The listing builds one solid part. Answer for the finished solid, in the listing's coordinates (mm). A direction names the side the tool comes from. Coordinates: 2 decimals unless noted, no trailing zeros. Order: outer loops, then holes, each group sorted by start corner. A loop starts at its lowest first (then second) coordinate and runs counter-clockwise, first axis right, second up. Notation, with made-up numbers: (52.5, -22) -> (62.5, -22) arc R9 ccw to (62.5, -8) -> close; hole circle Ø5 at (51.5, 25). An arc over 180 degrees is marked (long way). Put each result on its own line as item: value. Start each with the question number.
```python
from build123d import *

# Parameters (mm, degrees)
SKETCH1_R           = 19
SKETCH1_R_2         = 10.2
BOSS_EXTRUDE1_DEPTH = 5
SKETCH2_R           = 1.5
CUT_EXTRUDE1_DEPTH  = 5
BOSS_EXTRUDE2_START = -5
BOSS_EXTRUDE2_DEPTH = 5
SKETCH7_W           = 25
SKETCH7_H           = 5
BOSS_EXTRUDE5_DEPTH = 20
SKETCH8_W           = 20
SKETCH8_H           = 50
BOSS_EXTRUDE6_DEPTH = 5
SKETCH9_W           = 20
SKETCH9_H           = 50
BOSS_EXTRUDE7_DEPTH = 5


with BuildPart() as part:
    # Sketch1 → Boss-Extrude1 (new body)
    with BuildSketch(Plane(origin=(0, 0, 0), x_dir=(1, 0, 0), z_dir=(0, 1, 0))):
        with Locations(Location((0, 0, 0), (0, 0, 270))):
            Circle(SKETCH1_R)
        with Locations(Location((0, 0, 0), (0, 0, 270))):
            Circle(SKETCH1_R_2, mode=Mode.SUBTRACT)
    extrude(amount=BOSS_EXTRUDE1_DEPTH)

    # Sketch2 → Cut-Extrude1 (cut)
    with BuildSketch(Plane(origin=(0, 5, 0), x_dir=(1, 0, 0), z_dir=(0, 1, 0))):
        with Locations(Location((0, 14, 0), (0, 0, 270))):
            Circle(SKETCH2_R)
        with Locations(Location((7.5, 12.990381057, 0), (0, 0, 270))):
            Circle(SKETCH2_R)
        with Locations(Location((12.124355653, -7, 0), (0, 0, 270))):
            Circle(SKETCH2_R)
        with Locations(Location((7.5, -12.990381057, 0), (0, 0, 270))):
            Circle(SKETCH2_R)
        with Locations(Location((-12.124355653, -7, 0), (0, 0, 270))):
            Circle(SKETCH2_R)
        with Locations(Location((-15, 0, 0), (0, 0, 270))):
            Circle(SKETCH2_R)
    extrude(amount=-CUT_EXTRUDE1_DEPTH, mode=Mode.SUBTRACT)

    # Sketch3 → Boss-Extrude2 (add)
    with BuildSketch(Plane(origin=(0, 5, 0), x_dir=(1, 0, 0), z_dir=(0, 1, 0)).offset(BOSS_EXTRUDE2_START)):
        with BuildLine():
            ThreePointArc((19, 0), (13.435028843, -13.435028843), (0, -19))
            Line((0, -19), (23, -19))
            Line((23, -19), (23, 19))
            Line((23, 19), (0, 19))
            ThreePointArc((0, 19), (13.435028843, 13.435028843), (19, 0))
        make_face()
    extrude(amount=BOSS_EXTRUDE2_DEPTH)

    # Sketch7 → Boss-Extrude5 (add)
    with BuildSketch(Plane(origin=(23, 0, 0), x_dir=(0, 0, -1), z_dir=(1, 0, 0))):
        with Locations((0, 2.5)):
            Rectangle(SKETCH7_W, SKETCH7_H)
    extrude(amount=BOSS_EXTRUDE5_DEPTH)

    # Sketch8 → Boss-Extrude6 (add)
    with BuildSketch(Plane.XY.offset(12.5)):
        with Locations((33, -20)):
            Rectangle(SKETCH8_W, SKETCH8_H)
    extrude(amount=-BOSS_EXTRUDE6_DEPTH)

    # Sketch9 → Boss-Extrude7 (add)
    with BuildSketch(Plane(origin=(0, 0, -12.5), x_dir=(-1, 0, 0), z_dir=(0, 0, -1))):
        with Locations((-33, -20)):
            Rectangle(SKETCH9_W, SKETCH9_H)
    extrude(amount=-BOSS_EXTRUDE7_DEPTH)


solid = part.part
```
(1) For a pull along Z with two mould halves and no side action, classify faces 6 (the flat face through (11, 2, 19)), 7 (the cylindrical face through (6.587, 2.535, -14.181)), 8 (the flat face through (12, 2, -19)) as released by +Z, released by -Z, zero draft, split by the parting line, or undercut.
(2) Find the intervals of material crossed by L1, parallel to X at y = 2, z = 0; L2, parallel to Z at x = 39, y = -21; L3, parallel to X at y = 2.9, z = -14, in increasing order.
(3) A tool of negligible diameter and unlimited length cuts with its end or side. For faces 1 (the flat face through (33, -45, -10)), 2 (the cylindrical face through (-19, 2, 0)), 3 (the flat face through (33, -22, -7.5)), 4 (the flat face through (23, 2, -16)), 5 (the flat face through (23, -23, 10)), from which of +Z, -Z, +X, -X, +Y, -Y can it reach the whole face along a straight path? Write none if from no direction.
(4) The part is cut by section B-B on y = -41.5. Determine the outline of the cut face in (x, z).
(5) Each of these flat-tipped pins is pushed along its axis until it touches: P1, Ø5.5, axis at y = 2.5, z = 17, coming from the +X side; P2, Ø22, axis at x = 34, y = -30.5, coming from the -Z side; P3, Ø1.8, axis at x = 12.12, z = 7, coming from the +Y side; P4, Ø2.5, axis at y = -26.5, z = 9, coming from the -X side. Where does it stop, or does it pass through?
(6) The part is cut by section D-D on x = -15. Determine the outline of the cut face in (y, z).
(7) The part is cut by section C-C on z = 6.5. Determine the outline of the cut face in (x, y).
(8) The part is cut by section A-A on z = 0. Determine the outline of the cut face in (x, y).
Worked out:
1. face 6: released by +Z
1. face 7: undercut
1. face 8: released by -Z
2. L1: -19 to -16.5, -13.5 to -10.2, 10.2 to 43
2. L2: -12.5 to -7.5, 7.5 to 12.5
2. L3: -12.85 to -1.5, 1.5 to 6.39, 8.61 to 23
3. face 1: +Z, -Z, +X, -X, -Y
3. face 2: -X, +Y, -Y
3. face 3: +X, -X, -Y
3. face 4: -Z, +X, +Y, -Y
3. face 5: +Z, -Z, -X, -Y
4. outline: (23, -12.5) -> (43, -12.5) -> (43, -7.5) -> (23, -7.5) -> close; (23, 7.5) -> (43, 7.5) -> (43, 12.5) -> (23, 12.5) -> close
5. P1: x = 23
5. P2: z = -12.5
5. P3: through
5. P4: x = 23
6. outline: (0, -11.66) -> (5, -11.66) -> (5, -1.5) -> (0, -1.5) -> close; (0, 1.5) -> (5, 1.5) -> (5, 11.66) -> (0, 11.66) -> close
7. outline: (-17.85, 0) -> (-13.54, 0) -> (-13.54, 5) -> (-17.85, 5) -> close; (-10.71, 0) -> (-7.86, 0) -> (-7.86, 5) -> (-10.71, 5) -> close; (7.86, 0) -> (10.71, 0) -> (10.71, 5) -> (7.86, 5) -> close; (13.54, 0) -> (43, 0) -> (43, 5) -> (13.54, 5) -> close
8. outline: (-19, 0) -> (-16.5, 0) -> (-16.5, 5) -> (-19, 5) -> close; (-13.5, 0) -> (-10.2, 0) -> (-10.2, 5) -> (-13.5, 5) -> close; (10.2, 0) -> (43, 0) -> (43, 5) -> (10.2, 5) -> close
